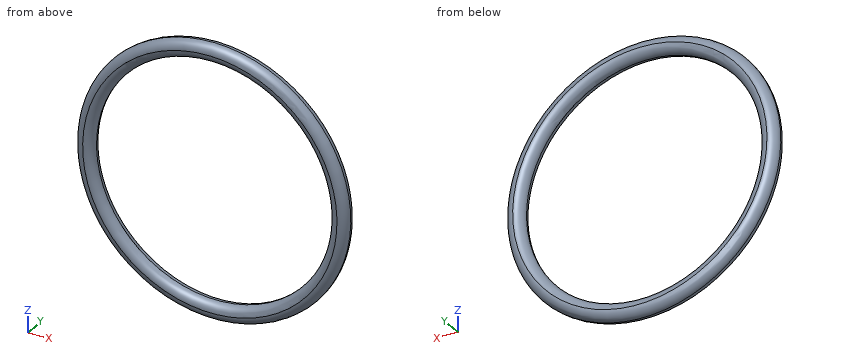
from build123d import *

# Parameters (mm, degrees)
SKETCH_2_R      = 23.5
SKETCH_2_R_2    = 20.5
EXTRUDE_1_DEPTH = 3
FILLET_2_R      = 1.5


with BuildPart() as part:
    # 草图2 → 凸台-拉伸1 (new body)
    with BuildSketch(Plane(origin=(0, 0, 0), x_dir=(1, 0, 0), z_dir=(0, 1, 0))):
        with Locations(Location((0, 0, 0), (0, 0, 270))):
            Circle(SKETCH_2_R)
        with Locations(Location((0, 0, 0), (0, 0, 270))):
            Circle(SKETCH_2_R_2, mode=Mode.SUBTRACT)
    extrude(amount=EXTRUDE_1_DEPTH)

    # 圆角2
    fillet_2_edges = [part.edges().sort_by_distance(p)[0] for p in [
        (0, 0, -23.5),
        (0, 3, -23.5),
        (0, 0, -20.5),
        (0, 3, -20.5),
    ]]
    fillet(fillet_2_edges, radius=FILLET_2_R - 0.0001)  # a hair under: the kernel refuses the full size


solid = part.part
The listing builds one solid part. Answer for the finished solid, in the listing's coordinates (mm). Coordinates: 2 decimals unless noted, no trailing zeros. Order: outer loops, then holes, each group sorted by start corner. A loop starts at its lowest first (then second) coordinate and runs counter-clockwise, first axis right, second up.
Q1. Given P1, Ø1.5, axis at x = 0.5, y = 2.5, coming from the +Z side, flat-ended and moving along its own axis, determine where the tip first touches the part or whether it passes through.
Q2. A cutting plane is placed at C-C, the plane y = 0.7. Write down the section's boundary in (x, z).
Q3. Consider line 1 (X direction, y = 1.5, z = 0); line 2 (Y direction, x = -5.5, z = 21.5); line 3 (X direction, y = 1.25, z = 11). Determine where each line is inside the solid, lowest interval first.
Answers follow:
1. P1: stops at z = 23.47
2. outline: circle Ø46.54 at (0, 0); hole circle Ø41.46 at (0, 0)
3. line 1: x = -23.5 to -20.5, 20.5 to 23.5
3. line 2: y = 0.01 to 2.99
3. line 3: x = -20.74 to -17.32, 17.32 to 20.74
